from build123d import *

# Parameters (mm, degrees)
ESQUISSE1_W        = 1
ESQUISSE1_H        = 0.5
ESQUISSE1_H_2      = 1
BOSS_EXTRU_2_DEPTH = 3
ESQUISSE1_4_W      = 4
ESQUISSE1_4_H      = 4
ESQUISSE1_4_R      = 1.5
BOSS_EXTRU_3_DEPTH = 12


with BuildPart() as part:
    # Esquisse1 → Boss.-Extru.2 (new body)
    with BuildSketch(Plane(origin=(0, 0, 0), x_dir=(1, 0, 0), z_dir=(0, 1, 0))):
        Polygon((2, 0), (0, 0), (0, -35), (2, -35), (2, -31), (6, -31), (6, -35), (22, -35), (22, -31), (26, -31), (26, -35), (28, -35), (28, 0), (26, 0), (26, -4), (22, -4), (22, 0), (6, 0), (6, -4), (2, -4), align=None)
        with Locations((12.5, -28.922446553)):
            Rectangle(ESQUISSE1_W, ESQUISSE1_H, mode=Mode.SUBTRACT)
        with Locations((6.5, -19.5)):
            Rectangle(ESQUISSE1_W, ESQUISSE1_H_2, mode=Mode.SUBTRACT)
        with Locations((9.5, -19.5)):
            Rectangle(ESQUISSE1_W, ESQUISSE1_H_2, mode=Mode.SUBTRACT)
        with Locations((12.5, -19.5)):
            Rectangle(ESQUISSE1_W, ESQUISSE1_H_2, mode=Mode.SUBTRACT)
        with Locations((14.5, -28.922446553)):
            Rectangle(ESQUISSE1_W, ESQUISSE1_H, mode=Mode.SUBTRACT)
        with Locations((16.5, -28.922446553)):
            Rectangle(ESQUISSE1_W, ESQUISSE1_H, mode=Mode.SUBTRACT)
        with Locations((15.5, -19.5)):
            Rectangle(ESQUISSE1_W, ESQUISSE1_H_2, mode=Mode.SUBTRACT)
        with Locations((18.5, -19.5)):
            Rectangle(ESQUISSE1_W, ESQUISSE1_H_2, mode=Mode.SUBTRACT)
        with Locations((21.5, -19.5)):
            Rectangle(ESQUISSE1_W, ESQUISSE1_H_2, mode=Mode.SUBTRACT)
    extrude(amount=BOSS_EXTRU_2_DEPTH)

    # Esquisse1_4 → Boss.-Extru.3 (add)
    # profile 1 of 4: a face of its own
    with BuildSketch(Plane(origin=(0, 0, 0), x_dir=(1, 0, 0), z_dir=(0, 1, 0))):
        with Locations((4, -2)):
            Rectangle(ESQUISSE1_4_W, ESQUISSE1_4_H)
        with Locations(Location((4, -1.7, 0), (0, 0, 270))):
            Circle(ESQUISSE1_4_R, mode=Mode.SUBTRACT)
    # profile 2 of 4: a face of its own
    with BuildSketch(Plane(origin=(0, 0, 0), x_dir=(1, 0, 0), z_dir=(0, 1, 0))):
        with Locations((4, -33)):
            Rectangle(ESQUISSE1_4_W, ESQUISSE1_4_H)
    # profile 3 of 4: a face of its own
    with BuildSketch(Plane(origin=(0, 0, 0), x_dir=(1, 0, 0), z_dir=(0, 1, 0))):
        with Locations((24, -2)):
            Rectangle(ESQUISSE1_4_W, ESQUISSE1_4_H)
        with Locations(Location((24, -1.7, 0), (0, 0, 270))):
            Circle(ESQUISSE1_4_R, mode=Mode.SUBTRACT)
    # profile 4 of 4: a face of its own
    with BuildSketch(Plane(origin=(0, 0, 0), x_dir=(1, 0, 0), z_dir=(0, 1, 0))):
        with Locations((24, -33)):
            Rectangle(ESQUISSE1_4_W, ESQUISSE1_4_H)
    extrude(amount=BOSS_EXTRU_3_DEPTH)


solid = part.part
Design review of the part built by this model. Coordinates are the model's own, in mm. A direction names the side the tool comes from. Coordinates: 2 decimals unless noted, no trailing zeros. Order: outer loops, then holes, each group sorted by start corner. A loop starts at its lowest first (then second) coordinate and runs counter-clockwise, first axis right, second up. Notation, with made-up numbers: M 79,10 L 87,10 A26 cw 87,29 Z; hole C 72,19.25 d4. An arc over 180 degrees is marked long. Use a Markdown table: item, result.
(1) Add section D-D (x = 12.5). Give the boundary of the cut face in (y, z), then the cut area to 4 significant figures.
Worked answers:
| item | result |
|---|---|
| outline | M 0,0 L 3,0 L 3,19 L 0,19 Z; M 0,20 L 3,20 L 3,28.67 L 0,28.67 Z; M 0,29.17 L 3,29.17 L 3,35 L 0,35 Z |
| area | 100.5 mm2 |
(2) For P1, Ø10, axis at x = 14, z = 17.5, coming from the +Y side; P2, Ø1.2, axis at y = 8, z = 32, coming from the +X side; P3, Ø3, axis at y = 6.5, z = 32, coming from the -X side; P4, Ø6, axis at x = 10, z = 15.5, coming from the -Y side, all flat-tipped, find the tip position at first contact; note any pin that passes through.
Worked answers:
| item | result |
|---|---|
| P1 | stops at y = 3 |
| P2 | stops at x = 26 |
| P3 | stops at x = 2 |
| P4 | stops at y = 0 |
(3) Draft analysis for pull direction Z (two halves, no side actions). For faces 1 (the flat face through (14, 2, 0)), 2 (the flat face through (19, 1.5, 19.5)), 3 (the flat face through (6, 7, 2)), state which applies: released by +Z, released by -Z, zero draft, split by the parting line, or undercut.
Worked answers:
| item | result |
|---|---|
| face 1 | released by -Z |
| face 2 | undercut |
| face 3 | zero draft |
(4) Add section B-B (x = 24). Give the boundary of the cut face in (y, z), then the cut area to 3 significant figures.
Worked answers:
| item | result |
|---|---|
| outline | M 0,0 L 12,0 L 12,0.2 L 0,0.2 Z; M 0,3.2 L 12,3.2 L 12,4 L 3,4 L 3,31 L 12,31 L 12,35 L 0,35 Z |
| area | 141 mm2 |
(5) Add section C-C (z = 1.7). Give the boundary of the cut face in (x, y), then the cut area to 3 significant figures.
Worked answers:
| item | result |
|---|---|
| outline | M 0,0 L 2.5,0 L 2.5,12 L 2,12 L 2,3 L 0,3 Z; M 5.5,0 L 22.5,0 L 22.5,12 L 22,12 L 22,3 L 6,3 L 6,12 L 5.5,12 Z; M 25.5,0 L 28,0 L 28,3 L 26,3 L 26,12 L 25.5,12 Z |
| area | 84.0 mm2 |
(6) Wall thickness on probe 1 along X at (y, z) = (2.75, 1.7); probe 2 along X at (y, z) = (6.75, 1.7); probe 3 along X at (y, z) = (9.25, 3.5): over which ranges is each line inside the solid? List them lowest first.
Worked answers:
| item | result |
|---|---|
| probe 1 | x = 0 to 2.5, 5.5 to 22.5, 25.5 to 28 |
| probe 2 | x = 2 to 2.5, 5.5 to 6, 22 to 22.5, 25.5 to 26 |
| probe 3 | x = 2 to 6, 22 to 26 |
(7) Add section A-A (y = 10.75). Give the boundary of the cut face in (x, z).
Worked answers:
| item | result |
|---|---|
| outline | M 2,0 L 6,0 L 6,4 L 2,4 Z; M 2,31 L 6,31 L 6,35 L 2,35 Z; M 22,0 L 26,0 L 26,4 L 22,4 Z; M 22,31 L 26,31 L 26,35 L 22,35 Z; hole C 4,1.7 d3; hole C 24,1.7 d3 |
(8) For faces 4 (the flat face through (12.5, 1.5, 20)), 5 (the flat face through (4, 7, 4)), 6 (the flat face through (6, 7, 33)), 7 (the flat face through (26, 7, 33)), list the 3-axis set-ups (+Z, -Z, +X, -X, +Y, -Y) from which the entire face can be reached by the end or side of a thin tool; tool diameter is ignored.
Worked answers:
| item | result |
|---|---|
| face 4 | +Y, -Y |
| face 5 | +X, -X, +Y |
| face 6 | +Z, -Z, +Y |
| face 7 | +Z, -Z, +X, +Y |
